Drawing for the job (mm, zero at the part's lowest x, y, z). A direction names the side the tool comes from. Coordinates: 2 decimals unless noted, no trailing zeros. Write each loop counter-clockwise with the first axis right and the second up, starting at its lowest first coordinate (ties: lowest second). Pieces come first, ordered by that corner, then holes. Notation, with made-up numbers: (9.5, 74.5) - (28.5, 74.5) arc R30 ccw to (28.5, 104.5) - close; hole circle Ø6 at (57.25, 44.5). An arc over 180 degrees is marked (long way). Write each question's results on one line, items separated by ' | '.
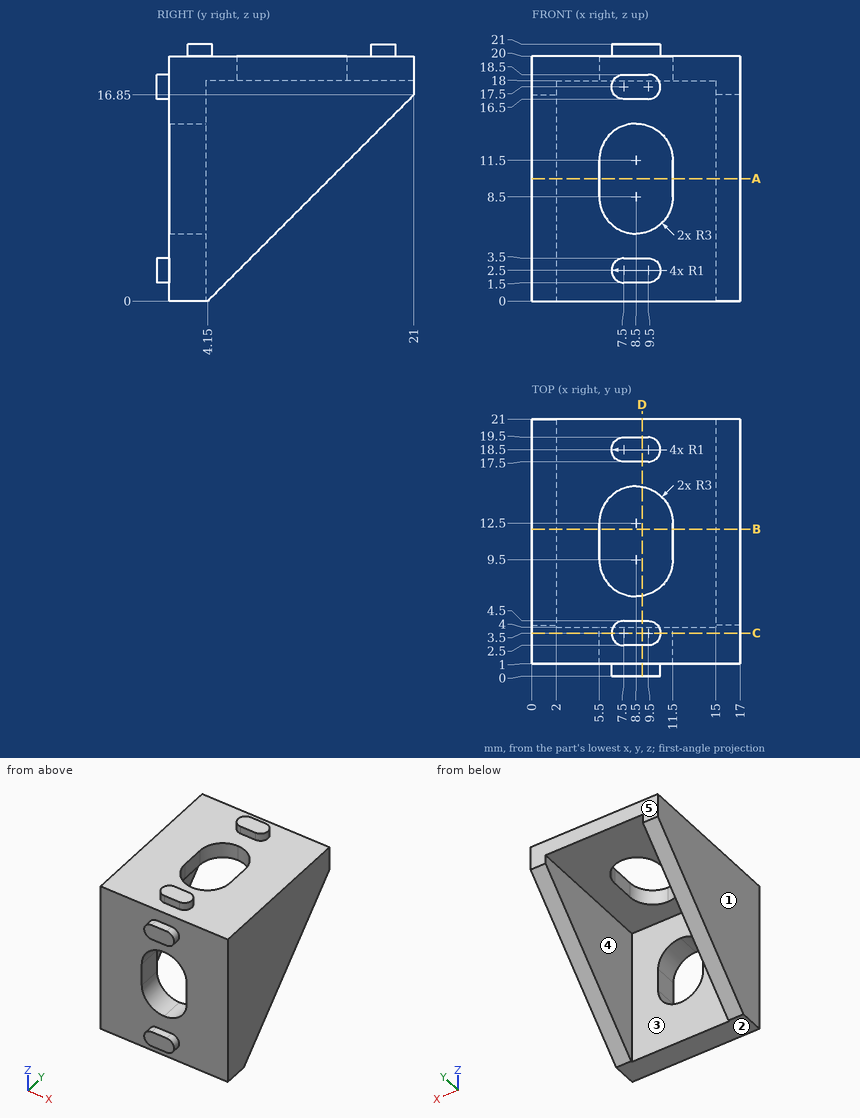
(1) Wall check: line 1 (X direction, y = 10, z = 11.5); line 2 (X direction, y = 11, z = 19.5); line 3 (Z direction, x = 2.5, y = 6). Give the ranges that are in metal, low to high. Write a range as from..to.
Return value:
line 1: x = 0..2, 15..17 | line 2: x = 0..5.5, 11.5..17 | line 3: z = 18..20
(2) Saw through at A-A on z = 10. Write the cut outline in (x, y), then the cut area to 3 significant figures.
Return value:
outline: (0, 1) - (5.5, 1) - (5.5, 4) - (2, 4) - (2, 14.15) - (0, 14.15) - close; (11.5, 1) - (17, 1) - (17, 14.15) - (15, 14.15) - (15, 4) - (11.5, 4) - close | area: 73.6 mm^2
(3) Flat gauge pins, fed straight in: P1, Ø4, axis at x = 15, y = 12.5, coming from the -Z side; P2, Ø8.5, axis at x = 8.5, y = 11, coming from the +Z side; P3, Ø5, axis at x = 10, z = 6.5, coming from the -Y side. Where does each tip first touch, or does it go through?
Return value:
P1: stops at z = 6.35 | P2: stops at z = 20 | P3: stops at y = 1
(4) Saw through at B-B on y = 12. Write the cut outline in (x, z), then the cut area to 3 significant figures.
Return value:
outline: (0, 7.85) - (2, 7.85) - (2, 18) - (5.5, 18) - (5.5, 20) - (0, 20) - close; (11.5, 18) - (15, 18) - (15, 7.85) - (17, 7.85) - (17, 20) - (11.5, 20) - close | area: 62.6 mm^2
(5) Saw through at C-C on y = 3.5. Write the cut outline in (x, z).
Return value:
outline: (0, 0) - (17, 0) - (17, 20) - (10.5, 20) - (10.5, 21) - (6.5, 21) - (6.5, 20) - (0, 20) - close; hole (5.5, 8.5) arc R3 ccw to (11.5, 8.5) - (11.5, 11.5) arc R3 ccw to (5.5, 11.5) - close
(6) Saw through at D-D on x = 9. Count the separate pieces of the cut face and the enclosed holes in it, then the cut area to 3 significant figures.
Return value:
separate pieces: 3 | enclosed holes: 0 | area: 57.4 mm^2
(7) Two-plate mould, pull along X, no slides. Class the marked faces 1, 2 and 3: released by +X, released by -X, zero draft, split by the parting line, or undercut.
Return value:
face 1: released by -X | face 2: zero draft | face 3: undercut
(8) 3-axis set-ups, long thin cutter, end or side, ignore diameter. For the marked faces 4 and 5: which of +Z, -Z, +X, -X, +Y, -Y reach the whole face in a straight line?
Return value:
face 4: -Z, +Y | face 5: +Z, -Z, +X, -X, +Y
